Geometry check sheet. Reference: the model listing, model coordinates, mm. A direction names the side the tool comes from. Round coordinates to 2 decimals unless told otherwise and drop trailing zeros. Loops run counter-clockwise (first coordinate to the right, second up) from the corner with the lowest first, then second, coordinate; pieces in that order, holes last.
```python
from build123d import *

# Parameters (mm, degrees)
SWEEP_THIN1_PROFILE_R   = 30
SWEEP_THIN1_PROFILE_R_2 = 20
SKETCH3_R               = 20
CUT_EXTRUDE1_DEPTH      = 1227.693525611
CUT_EXTRUDE1_DEPTH_BACK = 1227.693525611
SKETCH5_R               = 20
CUT_EXTRUDE3_DEPTH      = 111


with BuildPart() as part:
    # Sweep-Thin1: sweep along a path in Sketch1
    with BuildLine(Plane(origin=(0, 0, 0), x_dir=(0, 0, -1), z_dir=(1, 0, 0))) as sweep_thin1_path:
        Line((-41.871921182, 668.251231527), (108.128078818, 668.251231527))
        ThreePointArc((108.128078818, 668.251231527), (178.838756936, 638.961909646), (208.128078818, 568.251231527))
        Line((208.128078818, 568.251231527), (208.128078818, -91.748768473))
        Line((208.128078818, -91.748768473), (1008.128078818, -91.748768473))
    # Sweep-Thin1 profile (on start of the path) → Sweep-Thin1 (sweep)
    with BuildSketch(Plane(origin=(0, 668.251231527, 41.871921182), x_dir=(-1, 0, 0), z_dir=(0, 0, -1))):
        Circle(SWEEP_THIN1_PROFILE_R)
        Circle(SWEEP_THIN1_PROFILE_R_2, mode=Mode.SUBTRACT)
    sweep(path=sweep_thin1_path.line, transition=Transition.RIGHT)

    # Sketch3 → Cut-Extrude1 (cut, two sides)
    with BuildSketch(Plane(origin=(0, 0, 0), x_dir=(0, 0, -1), z_dir=(1, 0, 0))) as cut_extrude1_sk:
        with Locations(Location((208.128078818, -91.748768473, 0), (0, 0, 44.999997915))):
            Circle(SKETCH3_R)
    extrude(amount=CUT_EXTRUDE1_DEPTH, mode=Mode.SUBTRACT)
    extrude(cut_extrude1_sk.sketch, amount=-CUT_EXTRUDE1_DEPTH_BACK, mode=Mode.SUBTRACT)

    # Sketch5 → Cut-Extrude3 (cut)
    with BuildSketch(Plane.XY.offset(-330)):
        with Locations(Location((0, 383.251231527, 0), (0, 0, 270))):
            Circle(SKETCH5_R)
    extrude(amount=CUT_EXTRUDE3_DEPTH, mode=Mode.SUBTRACT)


solid = part.part
```
1) Sectioned sample at A-A, the plane y = -6.5. Record the cut outline in (x, z), then the cut area to 3 significant figures.
Report:
outline: circle Ø60 at (0, -208.13); hole circle Ø40 at (0, -208.13)
area: 1,570 mm2
2) Sectioned sample at B-B, the plane z = -917. Record the cut outline in (x, y), then the cut area to 3 significant figures.
Report:
outline: circle Ø60 at (0, -91.75); hole circle Ø40 at (0, -91.75)
area: 1,570 mm2
3) Scan lines: line 1 along Y through (x, z) = (1.5, -749); line 2 along Y through (x, z) = (0, 1); line 3 along Z through (x, y) = (1.5, 100.5). Record each from-to range of solid material in increasing order.
Report:
line 1: y = -121.71 to -111.69, -71.81 to -61.79
line 2: y = 638.25 to 648.25, 688.25 to 698.25
line 3: z = -238.09 to -228.07, -188.18 to -178.17
4) Mould release check, pull along X, two halves, no side actions. Record for faces 1 (the face through (2.6, -71.92, -613.73)), 2 (the face through (-20, 662, 41.872)), 3 (the face through (3.905, 697.996, -34.178)): +X half, -X half, draft (parallel to the pull), parting line (faces both ways), or undercut.
Report:
face 1: undercut
face 2: draft
face 3: parting line
5) Gauge pin test, flat ends, axial feed: pin 1 (6 mm diameter, centred on x = -10.5, z = -792, fed in from +Y); pin 2 (3 mm diameter, centred on x = 11, y = 263.5, fed in from -Z); pin 3 (8 mm diameter, centred on x = -6.5, z = -215, fed in from +Y). Record the tip position at first contact, or that the pin passes through.
Report:
pin 1: stops at y = -62.7
pin 2: stops at z = -236.58
pin 3: stops at y = 646.73
6) Access from +Z, -Z, +X, -X, +Y, -Y to the whole of each face (thin tool, end or side, straight path). Record for faces 4 (the face through (6.5, 218.42, -178.84)), 5 (the face through (-18.12, -105.26, -193.38)), 6 (the face through (4.336, 648.727, -34.178)), 7 (the face through (6.503, -121.035, -598.938)).
Report:
face 4: none
face 5: +X, -X
face 6: +Z
face 7: -Z
